```python
from build123d import *

# Parameters (mm, degrees)
SKETCH1_R                                      = 1.25
BOSS_EXTRUDE1_DEPTH                            = 2
CSK_FOR_M2_FLAT_HEAD_MACHINE_SCREW1_AT_2_COUNT = 2
CSK_FOR_M2_FLAT_HEAD_MACHINE_SCREW1_AT_2_PITCH = 41.6
CSK_FOR_M2_FLAT_HEAD_MACHINE_SCREW1_AT_3_COUNT = 2
CSK_FOR_M2_FLAT_HEAD_MACHINE_SCREW1_AT_3_PITCH = 48.126915546
CSK_FOR_M2_FLAT_HEAD_MACHINE_SCREW1_AT_4_COUNT = 2
CSK_FOR_M2_FLAT_HEAD_MACHINE_SCREW1_AT_4_PITCH = 24.2


with BuildPart() as part:
    # Sketch1 → Boss-Extrude1 (new body)
    with BuildSketch(Plane.XY):
        with BuildLine():
            Line((-28.8, 2.25), (-28.8, -2.25))
            Line((-28.8, -2.25), (-28.8, -2.75))
            ThreePointArc((-28.8, -2.75), (-28.433883476, -3.633883476), (-27.55, -4))
            Line((-27.55, -4), (-25.05, -4))
            ThreePointArc((-25.05, -4), (-24.166116524, -4.366116524), (-23.8, -5.25))
            Line((-23.8, -5.25), (-23.8, -12.1))
            ThreePointArc((-23.8, -12.1), (-20.8, -15.1), (-17.8, -12.1))
            Line((-17.8, -12.1), (-17.8, -11))
            Line((-17.8, -11), (17.8, -11))
            Line((17.8, -11), (17.8, -12.1))
            ThreePointArc((17.8, -12.1), (20.8, -15.1), (23.8, -12.1))
            Line((23.8, -12.1), (23.8, 12.1))
            ThreePointArc((23.8, 12.1), (20.8, 15.1), (17.8, 12.1))
            Line((17.8, 12.1), (17.8, 11))
            Line((17.8, 11), (-17.8, 11))
            Line((-17.8, 11), (-17.8, 12.1))
            ThreePointArc((-17.8, 12.1), (-20.8, 15.1), (-23.8, 12.1))
            Line((-23.8, 12.1), (-23.8, 5.25))
            ThreePointArc((-23.8, 5.25), (-24.166116524, 4.366116524), (-25.05, 4))
            Line((-25.05, 4), (-27.55, 4))
            ThreePointArc((-27.55, 4), (-28.433883476, 3.633883476), (-28.8, 2.75))
            Line((-28.8, 2.75), (-28.8, 2.25))
        make_face()
        with Locations((-20.8, 12.1)):
            Circle(SKETCH1_R, mode=Mode.SUBTRACT)
        with Locations((20.8, 12.1)):
            Circle(SKETCH1_R, mode=Mode.SUBTRACT)
        with Locations((20.8, -12.1)):
            Circle(SKETCH1_R, mode=Mode.SUBTRACT)
        with Locations((-20.8, -12.1)):
            Circle(SKETCH1_R, mode=Mode.SUBTRACT)
    extrude(amount=BOSS_EXTRUDE1_DEPTH)

    # Sketch3 → CSK for M2 Flat Head Machine Screw1 (revolve, cut)
    with BuildSketch(Plane(origin=(-20.8, 12.1, 2), x_dir=(0, -1, 0), z_dir=(1, 0, 0))):
        Polygon((0, 0), (0, 4.400860619), (1, 3.8), (1, 1.25), (2, 0.25), (2, 0), align=None)
    csk_for_m2_flat_head_machine_screw1 = revolve(axis=Axis((-20.8, 12.1, 8.35), (0, 0, -1)), mode=Mode.SUBTRACT)

    # CSK for M2 Flat Head Machine Screw1 at 2: CSK for M2 Flat Head Machine Screw1 ×2
    with Locations(*[(i * CSK_FOR_M2_FLAT_HEAD_MACHINE_SCREW1_AT_2_PITCH, 0, 0) for i in range(1, CSK_FOR_M2_FLAT_HEAD_MACHINE_SCREW1_AT_2_COUNT)]):
        add(csk_for_m2_flat_head_machine_screw1, mode=Mode.SUBTRACT)

    # CSK for M2 Flat Head Machine Screw1 at 3: CSK for M2 Flat Head Machine Screw1 ×2
    with Locations(*[Vector(0.864381179, -0.502837128, 0) * (i * CSK_FOR_M2_FLAT_HEAD_MACHINE_SCREW1_AT_3_PITCH) for i in range(1, CSK_FOR_M2_FLAT_HEAD_MACHINE_SCREW1_AT_3_COUNT)]):
        add(csk_for_m2_flat_head_machine_screw1, mode=Mode.SUBTRACT)

    # CSK for M2 Flat Head Machine Screw1 at 4: CSK for M2 Flat Head Machine Screw1 ×2
    with Locations(*[(0, -i * CSK_FOR_M2_FLAT_HEAD_MACHINE_SCREW1_AT_4_PITCH, 0) for i in range(1, CSK_FOR_M2_FLAT_HEAD_MACHINE_SCREW1_AT_4_COUNT)]):
        add(csk_for_m2_flat_head_machine_screw1, mode=Mode.SUBTRACT)


solid = part.part
```
The listing builds one solid part. Answer for the finished solid, in the listing's coordinates (mm). A direction names the side the tool comes from. Coordinates: 2 decimals unless noted, no trailing zeros. Write each loop counter-clockwise with the first axis right and the second up, starting at its lowest first coordinate (ties: lowest second). Pieces come first, ordered by that corner, then holes. Notation, with made-up numbers: (10, 40) - (25, 40) arc R17 ccw to (25, 47) - close; hole circle Ø3 at (-34, -1.5). An arc over 180 degrees is marked (long way). Return JSON: item names as keys, results as strings. Group by question number.
1. A cutting plane is placed at B-B, the plane y = 6.5. Determine the outline of the cut face in (x, z), plus the area to 3 significant figures.
2. A cutting plane is placed at A-A, the plane x = -20.8. Determine the outline of the cut face in (y, z).
3. Determine the mould class of faces 1 (the cylindrical face through (-28.424, 3.644, 0.986)), 2 (the flat face through (-3, 0, 0)), 3 (the cylindrical face through (-20.9, -15.1, 1)) for opening direction X: released by +X, released by -X, zero draft, split by the parting line, or undercut.
4. Given pin 1 (1.2 mm diameter, centred on y = 11.5, z = 1.5, fed in from -X); pin 2 (3 mm diameter, centred on x = 20.8, y = -12.1, fed in from +Z); pin 3 (1.5 mm diameter, centred on x = 20.8, y = 12.1, fed in from -Z); pin 4 (0.6 mm diameter, centred on x = -25.5, z = 0.5, fed in from +Y), each flat-ended and moving along its own axis, determine where each tip first touches the part or whether it passes through.
5. Straight lines are drawn through the part: L1, parallel to X at y = -12.1, z = 0.6; L2, parallel to Y at x = -20.8, z = 0.5; L3, parallel to X at y = 12.1, z = 1.9. For each, find the intervals that lie inside material, in ascending order.
6. A cutting plane is placed at C-C, the plane x = 6.5. Determine the outline of the cut face in (y, z).
7. Which of the six approach directions +Z, -Z, +X, -X, +Y, -Y give full straight-line access (tool end or side, diameter ignored) to faces 4 (the flat face through (23.8, 0, 1)), 5 (the flat face through (0, -11, 1)), 6 (the flat face through (-26, -4, 1))?
Ans:
{
 "1": {"outline": "(-23.8, 0) - (23.8, 0) - (23.8, 2) - (-23.8, 2) - close", "area": "95.2 mm²"},
 "2": {"outline": "(-15.1, 0) - (-13.35, 0) - (-13.35, 1) - (-14.1, 1.75) - (-14.1, 2) - (-15.1, 2) - close; (-10.85, 0) - (10.85, 0) - (10.85, 1) - (10.1, 1.75) - (10.1, 2) - (-10.1, 2) - (-10.1, 1.75) - (-10.85, 1) - close; (13.35, 0) - (15.1, 0) - (15.1, 2) - (14.1, 2) - (14.1, 1.75) - (13.35, 1) - close"},
 "3": {"face 1": "released by -X", "face 2": "zero draft", "face 3": "undercut"},
 "4": {"pin 1": "x = -23.8", "pin 2": "z = 1.25", "pin 3": "through", "pin 4": "y = 4"},
 "5": {"L1": "-23.8 to -22.05, -19.55 to -17.8, 17.8 to 19.55, 22.05 to 23.8", "L2": "-15.1 to -13.35, -10.85 to 10.85, 13.35 to 15.1", "L3": "-23.8 to -22.8, -18.8 to -17.8, 17.8 to 18.8, 22.8 to 23.8"},
 "6": {"outline": "(-11, 0) - (11, 0) - (11, 2) - (-11, 2) - close"},
 "7": {"face 4": "+Z, -Z, +X, +Y, -Y", "face 5": "+Z, -Z, -Y", "face 6": "+Z, -Z, -X, -Y"}
}
